```python
from build123d import *

# Parameters (mm, degrees)
SKETCH1_R                  = 193.675
BOSS_EXTRUDE1_DEPTH        = 6.35
F_9_0_196_DIAMETER_HOLE1_D = 4.9784
SKETCH5_R                  = 82.55
CUT_EXTRUDE1_DEPTH         = 6.35
F_9_0_196_DIAMETER_HOLE2_D = 4.9784


with BuildPart() as part:
    # Sketch1 → Boss-Extrude1 (new body)
    with BuildSketch(Plane(origin=(0, 0, 0), x_dir=(0, 1, 0), z_dir=(0, 0, 1))):
        with Locations(Location((0, 0, 0), (0, 0, 270))):
            Circle(SKETCH1_R)
    extrude(amount=BOSS_EXTRUDE1_DEPTH)

    # #9 (0.196) Diameter Hole1 (through all)
    with Locations(Plane.XY.offset(6.35)):
        with Locations((-150.657762959, 86.9823), (-173.9646, 0), (-150.657762959, -86.9823), (-86.9823, -150.657762959), (0, -173.9646), (86.9823, -150.657762959), (150.657762959, -86.9823), (173.9646, 0), (150.657762959, 86.9823), (86.9823, 150.657762959), (0, 173.9646), (-86.9823, 150.657762959)):
            Hole(F_9_0_196_DIAMETER_HOLE1_D / 2)

    # Sketch5 → Cut-Extrude1 (cut)
    with BuildSketch(Plane.XY.offset(6.35)):
        Circle(SKETCH5_R)
    extrude(amount=-CUT_EXTRUDE1_DEPTH, mode=Mode.SUBTRACT)

    # #9 (0.196) Diameter Hole2 (through all)
    with Locations(Plane.XY.offset(6.35)):
        with Locations((101.6, 66.675), (101.6, 41.275), (101.6, -9.525), (101.6, -34.925), (-101.6, -34.925), (-101.6, -9.525), (-101.6, 41.275), (-101.6, 66.675)):
            Hole(F_9_0_196_DIAMETER_HOLE2_D / 2)


solid = part.part
```
Design review of the part built by this model. Coordinates are the model's own, in mm. Coordinates: 2 decimals unless noted, no trailing zeros. Write each loop counter-clockwise with the first axis right and the second up, starting at its lowest first coordinate (ties: lowest second). Pieces come first, ordered by that corner, then holes.
1) Add section C-C (z = 1). State how many separate pieces and enclosed holes the cut face has, plus the area to 3 significant figures.
2) Add section A-A (x = -31.5). Write out the cut boundary in (y, z).
3) Add section B-B (y = -46). Write out the cut boundary in (x, z).
4) To check wall thickness, follow L1, parallel to Y at x = 0, z = 4.5 (3 decimals); L2, parallel to Y at x = -101.6, z = 5; L3, parallel to X at y = 87.5, z = 1.75. State the ranges of each line that lie inside material, in increasing order.
5) Insertion check: pin 1 (2 mm diameter, centred on x = 112.5, z = 4.5, fed in from -Y); pin 2 (3 mm diameter, centred on y = -19.5, z = 5, fed in from -X). Each pin has a flat end and moves straight along its axis. Give the tip position at first contact, or say it passes through.
6) Mouldability with a two-part tool opening along X and no side actions: class faces 1 (the cylindrical face through (-41.98, -189.07, 3.13)), 2 (the flat face through (83, 3, 6.35)), 3 (the cylindrical face through (-17.895, -80.587, 3.219)) as +X half, -X half, draft (parallel to the pull), parting line (faces both ways), or undercut.
Check result:
1. separate pieces: 1
1. enclosed holes: 21
1. area: 96,000 mm2
2. outline: (-191.1, 0) - (-76.3, 0) - (-76.3, 6.35) - (-191.1, 6.35) - close; (76.3, 0) - (191.1, 0) - (191.1, 6.35) - (76.3, 6.35) - close
3. outline: (-188.13, 0) - (-68.55, 0) - (-68.55, 6.35) - (-188.13, 6.35) - close; (68.55, 0) - (188.13, 0) - (188.13, 6.35) - (68.55, 6.35) - close
4. L1: y = -193.675 to -176.454, -171.475 to -82.55, 82.55 to 171.475, 176.454 to 193.675
4. L2: y = -164.89 to -37.41, -32.44 to -12.01, -7.04 to 38.79, 43.76 to 64.19, 69.16 to 164.89
4. L3: x = -172.78 to -153.09, -148.22 to 148.22, 153.09 to 172.78
5. pin 1: stops at y = -158.36
5. pin 2: stops at x = -192.84
6. face 1: parting line
6. face 2: draft
6. face 3: undercut
